Source: CAD feature listing. Evaluate the final solid. Frame: model axes, mm. Face numbers are marked on the shaded views. A direction names the side the tool comes from. Coordinates: 2 decimals unless noted, no trailing zeros. Loops run counter-clockwise (first coordinate to the right, second up) from the corner with the lowest first, then second, coordinate; pieces in that order, holes last.
Item 1: Reachability of the marked faces 4 and 5 from +Z, -Z, +X, -X, +Y, -Y: full face, straight path, thin tool, end or side. Return the list, or none.
Item 2: Section query D-D, the plane y = -4. Return the cut outline in (x, z), then the cut area to 3 significant figures.
Item 3: Pull-direction query (Y, two-part tool) for the marked faces 1, 2 and 3; classes: +Y half, -Y half, draft (parallel to the pull), parting line (faces both ways), or undercut.
Item 4: Section query C-C, the plane z = 4.1. State how many separate pieces and enclosed holes the cut face has, then the cut area to 3 significant figures.
Item 5: Section query A-A, the plane y = 64.1. Return the cut outline in (x, z).
Item 6: Line query: probe 1 along Y at (x, z) = (0, 3.6); probe 2 along Y at (x, z) = (-8.75, 1.5); probe 3 along X at (y, z) = (75.1, 1.95). Output: solid intervals per line, ascending.
Item 7: Section query B-B, the plane x = 0. Return the cut outline in (y, z), then the cut area to 3 significant figures.
Autodesk Inventor part; units mm, degrees
ref_plane "YZ Plane" through (0, 0, 0) normal (1, 0, 0) x (0, 1, 0)
ref_plane "XZ Plane" through (0, 0, 0) normal (0, 1, 0) x (-1, 0, 0)
ref_plane "XY Plane" through (0, 0, 0) normal (0, 0, 1) x (1, 0, 0)
sketch "스케치1" plane through (0, 0, 0) normal (0, 0, 1) x (1, 0, 0)
  circle A0 centre (0, 0) radius 13.8
  circle A1 centre (0, 0) radius 7.2
  circle A2 centre (0, -11) radius 1.2812
  circle A3 centre (-7.7782, -7.7782) radius 1.2812
  circle A4 centre (-11, 0) radius 1.2812
  circle A5 centre (-7.7782, 7.7782) radius 1.2812
  circle A6 centre (0, 11) radius 1.2812
  circle A7 centre (7.7782, 7.7782) radius 1.2812
  circle A8 centre (11, 0) radius 1.2812
  circle A9 centre (7.7782, -7.7782) radius 1.2812
  circle A10 centre (0, 75.1) radius 13.8
  circle A11 centre (0, 75.1) radius 7.2
  circle A12 centre (0, 64.1) radius 1.2812
  circle A13 centre (-7.7782, 67.3218) radius 1.2812
  circle A14 centre (-11, 75.1) radius 1.2812
  circle A15 centre (-7.7782, 82.8782) radius 1.2812
  circle A16 centre (0, 86.1) radius 1.2812
  circle A17 centre (7.7782, 82.8782) radius 1.2812
  circle A18 centre (11, 75.1) radius 1.2812
  circle A19 centre (7.7782, 67.3218) radius 1.2812
  circle A20 centre (7.7782, -7.7782) radius 3.8
  circle A21 centre (-7.7782, -7.7782) radius 3.8
  line L0 (-113.808, 75.1) -> (55.228, 75.1)
  line L1 (13.8, 0) -> (13.8, 75.1)
  line L2 (-13.8, 0) -> (-13.8, 75.1)
  circle A22 centre (7.7782, 82.8782) radius 3.8
  circle A23 centre (-7.7782, 82.8782) radius 3.8
  point P0 (0, 0)
  point P1 (5.0912, -5.0912)
  point P2 (7.5223, -11.5696)
  point P3 (7.5223, 86.6696)
  point P4 (5.0912, 80.1912)
  point P5 (-5.0912, 80.1912)
  point P6 (-7.5223, 86.6696)
  point P7 (-7.5223, -11.5696)
  point P8 (-5.0912, -5.0912)
extrude "돌출1" add sketch "스케치1" along normal blind 6 contours A0 A20 A1 A21 | A0 L2 A10 L1 | A0 A20 | L0 A18 A11 A22 A10 | A10 L0 A14 A11 A18 | A21 A0 | A10 A23 A11 L0 A14 | A22 A10 | A10 A23 picked at (4.2604, 10.6567) picked at (10.3474, -8.1187) picked at (-10.3474, -8.1187) picked at (10.3474, 83.2187) picked at (-10.3474, 83.2187)
properties part number "_shim"
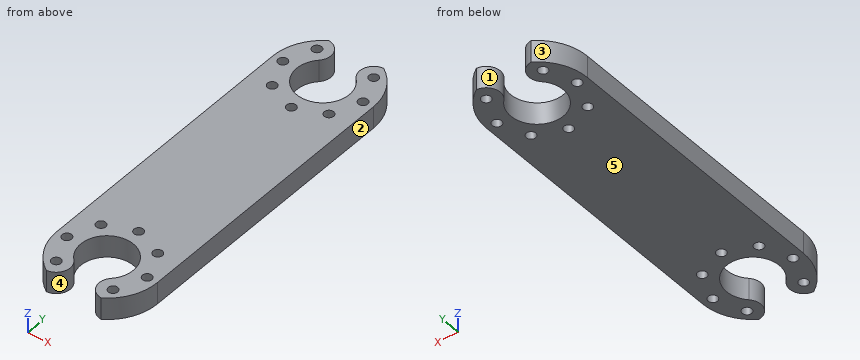
Verdict:
1. face 4: +Z, -Z
1. face 5: -Z, +X, -X, +Y, -Y
2. outline: (-13.21, 0) - (-5.99, 0) - (-5.99, 6) - (-13.21, 6) - close; (5.99, 0) - (13.21, 0) - (13.21, 6) - (5.99, 6) - close
2. area: 86.7 mm2
3. face 1: undercut
3. face 2: draft
3. face 3: +Y half
4. separate pieces: 1
4. enclosed holes: 14
4. area: 2,140 mm2
5. outline: (-13.8, 0) - (-1.28, 0) - (-1.28, 6) - (-13.8, 6) - close; (1.28, 0) - (13.8, 0) - (13.8, 6) - (1.28, 6) - close
6. probe 1: y = 7.2 to 9.72, 12.28 to 62.82, 65.38 to 67.9
6. probe 2: y = -10.67 to -8.61, -6.94 to 6.94, 8.61 to 66.49, 68.16 to 82.04, 83.71 to 85.77
6. probe 3: x = -13.8 to -12.28, -9.72 to -7.2, 7.2 to 9.72, 12.28 to 13.8
7. outline: (7.2, 0) - (9.72, 0) - (9.72, 6) - (7.2, 6) - close; (12.28, 0) - (62.82, 0) - (62.82, 6) - (12.28, 6) - close; (65.38, 0) - (67.9, 0) - (67.9, 6) - (65.38, 6) - close
7. area: 333 mm2
